Geometry: final body of the model. Coordinates: model frame, mm. Face numbers are marked on the shaded views. A direction names the side the tool comes from. Give positions to 0.01 mm unless a question says otherwise; leave off trailing zeros. Write each loop counter-clockwise with the first axis right and the second up, starting at its lowest first coordinate (ties: lowest second). Pieces come first, ordered by that corner, then holes. Notation, with made-up numbers: M -25,-17 L 15,-17 A35 ccw 15,15 Z; hole C 41,23.25 d1. An arc over 180 degrees is marked long. Answer as a JSON object with one key per item and string values.
from build123d import *

# Parameters (mm, degrees)
SKETCH1_W           = 50
SKETCH1_H           = 36
SKETCH1_R           = 1.55
SKETCH1_R_2         = 8
BOSS_EXTRUDE1_DEPTH = 4
SKETCH2_W           = 50
SKETCH2_H           = 4
BOSS_EXTRUDE3_DEPTH = 34
SKETCH3_W           = 29
SKETCH3_H           = 13
CUT_EXTRUDE1_DEPTH  = 67.80007485
BOSS_EXTRUDE4_DEPTH = 15
SKETCH7_W           = 50
SKETCH7_H           = 4
BOSS_EXTRUDE5_DEPTH = 15
SKETCH9_W           = 29
SKETCH9_H           = 6.5
CUT_EXTRUDE2_DEPTH  = 71.215738976
SKETCH10_R          = 2.65
CUT_EXTRUDE3_DEPTH  = 69.134059031


with BuildPart() as part:
    # Sketch1 → Boss-Extrude1 (new body)
    with BuildSketch(Plane(origin=(0, 0, 0), x_dir=(1, 0, 0), z_dir=(0, 1, 0))):
        with Locations((16.5, 9)):
            Rectangle(SKETCH1_W, SKETCH1_H)
        with Locations(Location((0, 18, 0), (0, 0, 270))):
            Circle(SKETCH1_R, mode=Mode.SUBTRACT)
        with Locations(Location((0, 0, 0), (0, 0, 270))):
            Circle(SKETCH1_R, mode=Mode.SUBTRACT)
        with Locations(Location((33, 0, 0), (0, 0, 270))):
            Circle(SKETCH1_R, mode=Mode.SUBTRACT)
        with Locations(Location((33, 18, 0), (0, 0, 270))):
            Circle(SKETCH1_R, mode=Mode.SUBTRACT)
        with Locations(Location((9, 9, 0), (0, 0, 270))):
            Circle(SKETCH1_R_2, mode=Mode.SUBTRACT)
    extrude(amount=BOSS_EXTRUDE1_DEPTH)

    # Sketch2 → Boss-Extrude3 (add)
    with BuildSketch(Plane(origin=(0, 4, 0), x_dir=(1, 0, 0), z_dir=(0, 1, 0))):
        with Locations((16.5, -7)):
            Rectangle(SKETCH2_W, SKETCH2_H)
        with Locations((16.5, 25)):
            Rectangle(SKETCH2_W, SKETCH2_H)
    extrude(amount=BOSS_EXTRUDE3_DEPTH)

    # Sketch3 → Cut-Extrude1 (cut, through all)
    with BuildSketch(Plane.XY.offset(9)):
        with Locations((16.5, 31.5)):
            Rectangle(SKETCH3_W, SKETCH3_H)
    extrude(amount=-CUT_EXTRUDE1_DEPTH, mode=Mode.SUBTRACT)

    # Sketch6 → Boss-Extrude4 (add)
    with BuildSketch(Plane.XY.offset(9)):
        Polygon((31, 38), (41.5, 38), (41.5, 34), (2, 34), (-8.5, 34), (-8.5, 38), align=None)
    extrude(amount=BOSS_EXTRUDE4_DEPTH)

    # Sketch7 → Boss-Extrude5 (add)
    with BuildSketch(Plane(origin=(0, 0, -27), x_dir=(-1, 0, 0), z_dir=(0, 0, -1))):
        with Locations((-16.5, 36)):
            Rectangle(SKETCH7_W, SKETCH7_H)
    extrude(amount=BOSS_EXTRUDE5_DEPTH)

    # Sketch9 → Cut-Extrude2 (cut, through all)
    with BuildSketch(Plane(origin=(0, 38, 0), x_dir=(1, 0, 0), z_dir=(0, 1, 0))):
        with Locations((16.5, 30.25)):
            Rectangle(SKETCH9_W, SKETCH9_H)
        with Locations((16.5, -12.25)):
            Rectangle(SKETCH9_W, SKETCH9_H)
    extrude(amount=-CUT_EXTRUDE2_DEPTH, mode=Mode.SUBTRACT)

    # Sketch10 → Cut-Extrude3 (cut, through all)
    with BuildSketch(Plane.XZ.offset(-34)):
        with Locations(Location((36.5, -36, 0), (0, 0, 270))):
            Circle(SKETCH10_R)
        with Locations(Location((-3.5, -36, 0), (0, 0, 270))):
            Circle(SKETCH10_R)
        with Locations(Location((-3.5, 18, 0), (0, 0, 270))):
            Circle(SKETCH10_R)
        with Locations(Location((36.5, 18, 0), (0, 0, 270))):
            Circle(SKETCH10_R)
    extrude(amount=-CUT_EXTRUDE3_DEPTH, mode=Mode.SUBTRACT)


solid = part.part
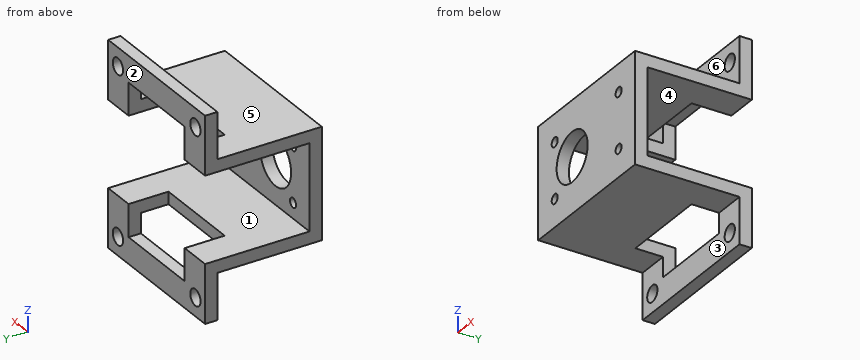
1) Line query: line 1 (X direction, y = 35.65, z = 18); line 2 (X direction, y = 1.9, z = 0); line 3 (Z direction, x = -2, y = 10.5). Output: solid intervals per line, ascending. Write a range as from..to.
Geometry check:
{"line 1": "x = -8.5..-6.15, -0.85..33.85, 39.15..41.5", "line 2": "x = -8.5..-1.55, 1.55..31.45, 34.55..41.5", "line 3": "z = -27..-23, 5..9"}
2) Set-up query: the marked faces 1, 2 and 3. Return all of +Z, -Z, +X, -X, +Y, -Y with unobstructed straight access to the full face (end or side cutting, diameter ignored); none if empty.
Geometry check:
{"face 1": "+X, -X, +Y", "face 2": "+Z, -Z, +X, -X, +Y", "face 3": "-Z, +X, -X, -Y"}
3) Cut plane D-D on y = 27. Return loops of the section in (x, z), and give its area (3 significant figures).
Geometry check:
{"outline": "M -8.5,-27 L 2,-27 L 2,-23 L -8.5,-23 Z; M -8.5,5 L 2,5 L 2,9 L -8.5,9 Z; M 31,-27 L 41.5,-27 L 41.5,-23 L 31,-23 Z; M 31,5 L 41.5,5 L 41.5,9 L 31,9 Z", "area": "168 mm2"}
4) Cut plane A-A on x = 9. Return loops of the section in (y, z).
Geometry check:
{"outline": "M 0,-27 L 25,-27 L 25,-23 L 4,-23 L 4,-17 L 0,-17 Z; M 0,-1 L 4,-1 L 4,5 L 25,5 L 25,9 L 0,9 Z; M 34,-42 L 38,-42 L 38,-33.5 L 34,-33.5 Z; M 34,15.5 L 38,15.5 L 38,24 L 34,24 Z"}
5) Pull-direction query (Z, two-part tool) for the marked faces 4, 5 and 6; classes: pulls with the +Z half, pulls with the -Z half, needs draft (parallel to the pull), parting line crosses it, or undercut.
Geometry check:
{"face 4": "undercut", "face 5": "pulls with the +Z half", "face 6": "needs draft"}
6) Cut plane C-C on z = -9. Return loops of the section in (x, y).
Geometry check:
{"outline": "M -8.5,0 L 1,0 L 1,4 L -8.5,4 Z; M 17,0 L 41.5,0 L 41.5,4 L 17,4 Z"}
7) Contact query for flat-ended pins moving along their axis: P1, Ø3, axis at y = 30, z = -30, coming from the -X side; P2, Ø6, axis at x = 36.5, z = -36, coming from the -Y side; P3, Ø2, axis at x = 21, z = 7, coming from the +Y side; P4, Ø2, axis at x = 19.5, y = 17.5, coming from the +Z side. Output: stop coordinate, or through.
Geometry check:
{"P1": "passes through", "P2": "stops at y = 34", "P3": "stops at y = 25", "P4": "stops at z = 9"}
8) Cut plane B-B on y = 22. Return loops of the section in (x, z), and give its area (3 significant figures).
Geometry check:
{"outline": "M -8.5,-27 L 41.5,-27 L 41.5,-23 L -8.5,-23 Z; M -8.5,5 L 41.5,5 L 41.5,9 L -8.5,9 Z", "area": "400 mm2"}
